Autodesk Inventor part; units mm, degrees
ref_plane "YZ Plane" through (0, 0, 0) normal (1, 0, 0) x (0, 1, 0)
ref_plane "XZ Plane" through (0, 0, 0) normal (0, 1, 0) x (-1, 0, 0)
ref_plane "XY Plane" through (0, 0, 0) normal (0, 0, 1) x (1, 0, 0)
sketch "Эскиз1" plane through (0, 0, 0) normal (0, 0, 1) x (1, 0, 0)
  line L0 (-60, 0) -> (60, 0)
  line L1 (60, 0) -> (60, 5)
  line L2 (60, 5) -> (-60, 5)
  line L3 (-60, 5) -> (-60, 0)
  point P0 (0, 0)
  point P1 (0, 0)
  dimension "d0" = 5
  dimension "d1" = 120
extrude "Выдавливание1" add sketch "Эскиз1" along normal mid plane 20
sketch "Эскиз3" plane through (0, 0, 0) normal (0, 0, 1) x (1, 0, 0)
  line L0 (-60, 5) -> (-58.5441, 9)
  line L1 (-58.5441, 9) -> (-57.5, 9)
  line L2 (-57.5, 9) -> (-56.0441, 5)
  line L3 (-60, 5) -> (60, 5)
  line L4 (-59.2721, 7) -> (-56.7721, 7) construction
  point P0 (0, 0)
  dimension "d4" = 40
  dimension "d5" = 4
  dimension "d6" = 2.5
extrude "Выдавливание2" add sketch "Эскиз3" against normal up to surface (20 mm away) from surface at 10
pattern_linear "Прямоуг.массив1" count 20 spacing 5 along (1, 0, 0) of "Выдавливание2"
properties part number "rack"
Design review of the part built by this model. Coordinates are the model's own, in mm. A direction names the side the tool comes from. Coordinates: 2 decimals unless noted, no trailing zeros. Answer as a JSON object with one key per item and string values. Group by question number.
1) Add section A-A, the plane y = 6. Count the separate pieces of the cut face and the enclosed holes in it, then the cut area to 3 significant figures.
2) For pin 1 (0.8 mm diameter, centred on x = -50.5, z = -1, fed in from +Y), flat-tipped, find the tip position at first contact; note if it passes through.
3) Tool access review of faces 4 (the flat face through (-9.282, 6.972, 0.14)), 5 (the flat face through (-1, 4, 10)): name each direction out of +Z, -Z, +X, -X, +Y, -Y from which nothing blocks a thin tool from reaching the whole face with its end or side.
4) Wall thickness on L1, parallel to Y at x = -36, z = -8.25: over which ranges is the line inside the solid? List them lowest first.
5) Mouldability with a two-part tool opening along X and no side actions: class faces 1 (the flat face through (-41.782, 7.028, 0.14)), 2 (the flat face through (-1, 4, -10)), 3 (the flat face through (-60, 3, 0)) as pulls with the +X half, pulls with the -X half, needs draft (parallel to the pull), parting line crosses it, or undercut.
Computed values:
{
 "1": {"separate pieces": "20", "enclosed holes": "0", "area": "1,290 mm^2"},
 "2": {"pin 1": "stops at y = 5"},
 "3": {"face 4": "+Z, -Z, +Y", "face 5": "+Z, +X, -X, +Y, -Y"},
 "4": {"L1": "y = 0 to 5"},
 "5": {"face 1": "undercut", "face 2": "needs draft", "face 3": "pulls with the -X half"}
}
